Can you work these out from the model? Positions are in its coordinate system, mm. Face numbers are marked on the shaded views. A direction names the side the tool comes from. Coordinates: 2 decimals unless noted, no trailing zeros. Loops run counter-clockwise (first coordinate to the right, second up) from the corner with the lowest first, then second, coordinate; pieces in that order, holes last. Notation, with made-up numbers: (-2, 35) -> (14, 35) arc R20 ccw to (14, 50) -> close; hole circle Ø3 at (26, 66). An arc over 180 degrees is marked (long way). Use one line per item in the form item = value. Start each with the question number.
(1) I need wall thicknesses on line 1 (Y direction, x = 0, z = 12); line 2 (Z direction, x = 2.25, y = 2). Which ranges of each line are inside material? Lowest first, please. Write a range as [from, to].
(2) On a 3-axis mill with a long thin cutter (end or side, diameter ignored), from which of +Z, -Z, +X, -X, +Y, -Y can I reach the whole of each face in a straight line? I mean the marked faces 1 and 2. Say none if no direction works.
(3) Imagine slicing it at A-A (z = 8). List the corners of the cut face in (x, y) for me, plus the area to 3 significant figures.
(4) I'm going to push flat-ended pins straight in: pin 1 (3.5 mm diameter, centred on x = 1.5, y = -1.5, fed in from +Z); pin 2 (3 mm diameter, centred on y = -0.5, z = 5.5, fed in from -X); pin 3 (1 mm diameter, centred on y = -2.5, z = 17.5, fed in from +X). Where does each tip first touch, or does it pass through?
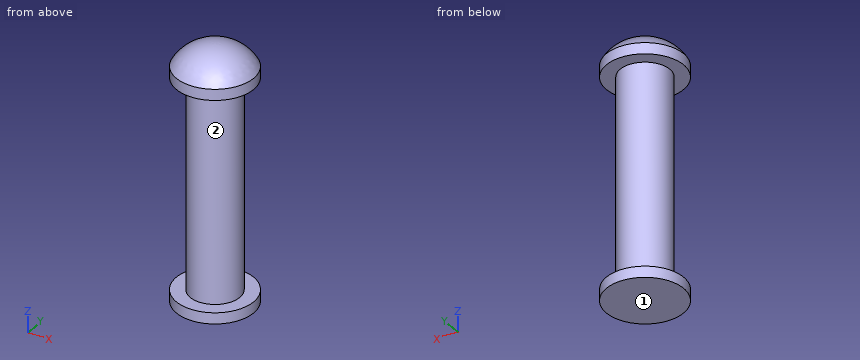
```python
from build123d import *

# Parameters (mm, degrees)
F0_R     = 2.25
F1_DEPTH = 20
F2_R     = 3.5
F3_DEPTH = 1
F4_R     = 3.5
F5_DEPTH = 1


with BuildPart() as f1:
    # F0 (on Top) → F1 (new body)
    with BuildSketch(Plane.XY):
        Circle(F0_R)
    extrude(amount=F1_DEPTH)

    # F2 (on face) → F3 (join)
    with BuildSketch(Plane(origin=(0, 0, 0), x_dir=(1, 0, 0), z_dir=(0, 0, -1))):
        Circle(F2_R)
    extrude(amount=-F3_DEPTH)

    # F4 (on face) → F5 (join)
    with BuildSketch(Plane.XY.offset(20)):
        Circle(F4_R)
    extrude(amount=F5_DEPTH)

    # F6 (on Front) → F7 (revolve)
    with BuildSketch(Plane.XZ):
        with BuildLine():
            Line((0, 20.991329), (0, 23))
            ThreePointArc((0, 23), (-2.022616, 22.477079), (-3.5, 21))
            Line((-3.5, 21), (0, 20.991329))
        make_face()
    revolve(axis=Axis((0, 0, 11.212396), (0, 0, 1)))


solid = f1.part
```
Worked out:
q1.line_1 = [-2.25, 2.25]
q1.line_2 = [0, 1], [20, 21.68]
q2.face_1 = -Z, +X, -X, +Y, -Y
q2.face_2 = none
q3.outline = circle Ø4.5 at (0, 0)
q3.area = 15.9 mm2
q4.pin_1 = 22.99
q4.pin_2 = -2.25
q4.pin_3 = 1.03
